from build123d import *

# Parameters (mm, degrees)
F1_DEPTH = 4
F0_W     = 28
F0_H     = 79
F2_DEPTH = 30
F3_W     = 10
F3_H     = 1.5
F4_DEPTH = 4
F6_DEPTH = 30
F5_W     = 20
F5_H     = 42
F7_DEPTH = 4
F8_R     = 5
F9_DEPTH = 4


with BuildPart() as f1:
    # F0 (on Top) → F1 (new body)
    with BuildSketch(Plane.XY):
        Polygon((17, 4), (24, 4), (24, 75), (4, 75), (4, 4), (11, 4), (11, 5.5), (14, 5.5), (17, 5.5), align=None)
    extrude(amount=F1_DEPTH)

    # F0 (on Top) → F2 (join)
    with BuildSketch(Plane.XY):
        with Locations((14, 39.5)):
            Rectangle(F0_W, F0_H)
        Polygon((24, 75), (24, 4), (17, 4), (14, 4), (11, 4), (4, 4), (4, 75), align=None, mode=Mode.SUBTRACT)
    extrude(amount=F2_DEPTH)

    # F3 (on face) → F4 (cut, through all)
    with BuildSketch(Plane(origin=(0, 79, 0), x_dir=(-1, 0, 0), z_dir=(0, 1, 0))):
        with Locations((-9, 29.25)):
            Rectangle(F3_W, F3_H)
        with Locations((-19, 29.25)):
            Rectangle(F3_W, F3_H)
    extrude(amount=-F4_DEPTH, mode=Mode.SUBTRACT)

    # F5 (on Top) → F6 (join)
    with BuildSketch(Plane.XY):
        Polygon((24, 79), (28, 79), (28, 125), (0, 125), (0, 79), (4, 79), (4, 121), (24, 121), align=None)
    extrude(amount=F6_DEPTH)

    # F5 (on Top) → F7 (join)
    with BuildSketch(Plane.XY):
        with Locations((14, 100)):
            Rectangle(F5_W, F5_H)
    extrude(amount=F7_DEPTH)

    # F8 (on face) → F9 (cut, through all)
    with BuildSketch(Plane(origin=(0, 125, 0), x_dir=(-1, 0, 0), z_dir=(0, 1, 0))):
        with Locations((-14, 15)):
            Circle(F8_R)
    extrude(amount=-F9_DEPTH, mode=Mode.SUBTRACT)


solid = f1.part
Model file for the job. Use its own axes, mm. A direction names the side the tool comes from. Give positions to 0.01 mm unless a question says otherwise; leave off trailing zeros. Order: outer loops, then holes, each group sorted by start corner. A loop starts at its lowest first (then second) coordinate and runs counter-clockwise, first axis right, second up. Notation, with made-up numbers: M 14.5,72.5 L 66.5,72.5 A25 ccw 66.5,97.5 Z; hole C 22,6 d7. An arc over 180 degrees is marked long. Put each result on its own line as item: value. Start each with the question number.
(1) Band-saw the part on D-D on z = 15. Give the cut face in (x, y).
(2) Band-saw the part on A-A on z = 21.75. Give the cut face in (x, y).
(3) Drill centre lines: L1, parallel to Y at x = 14.25, z = 8.25; L2, parallel to X at y = 12.5, z = 15.25; L3, parallel to Z at x = 14, y = 122.75. Where is each one in solid material? Low to high. Write a range as [from, to].
(4) Pin check, flat tips, straight feed: pin 1 Ø2 at (x, z) = (13.5, 17) entering from +Y; pin 2 Ø8 at (y, z) = (46, 12.5) entering from -X; pin 3 Ø4.5 at (x, y) = (14.5, 76) entering from +Z; pin 4 Ø3 at (x, y) = (16, 104.5) entering from +Z. Stop position of each tip, or through.
(5) Band-saw the part on C-C on y = 33.5. Give the cut face in (x, z).
(6) Tool access for faces 1 (the face through (0, 63, 15)), 2 (the face through (14, 5.5, 2)), 3 (the face through (14, 4, 15)): list every direction of +Z, -Z, +X, -X, +Y, -Y with a clear straight run to the whole face (end or side of a thin tool).
(7) Band-saw the part on B-B on x = 14. Give the cut face in (y, z).
(8) Pull direction Z, two halves, no side cores. Call faces 4 (the face through (11.693, 123.028, 10.564)), 5 (the face through (3.6, 58.2, 30)), 6 (the face through (14, 63, 0)), 7 (the face through (16, 121, 20)): released by +Z, released by -Z, zero draft, split by the parting line, or undercut.
Results below:
1. outline: M 0,0 L 28,0 L 28,125 L 19,125 L 19,121 L 24,121 L 24,79 L 4,79 L 4,121 L 9,121 L 9,125 L 0,125 Z; hole M 4,4 L 24,4 L 24,75 L 4,75 Z
2. outline: M 0,0 L 28,0 L 28,125 L 0,125 Z; hole M 4,4 L 24,4 L 24,75 L 4,75 Z; hole M 4,79 L 24,79 L 24,121 L 4,121 Z
3. L1: y = [0, 4], [75, 79], [121, 125]
3. L2: x = [0, 4], [24, 28]
3. L3: z = [0, 10], [20, 30]
4. pin 1: stops at y = 79
4. pin 2: stops at x = 0
4. pin 3: stops at z = 28.5
4. pin 4: stops at z = 4
5. outline: M 0,0 L 28,0 L 28,30 L 24,30 L 24,4 L 4,4 L 4,30 L 0,30 Z
6. face 1: +Z, -Z, -X, +Y, -Y
6. face 2: +Z, -Z
6. face 3: +Z
7. outline: M 0,0 L 4,0 L 4,30 L 0,30 Z; M 5.5,0 L 125,0 L 125,10 L 121,10 L 121,4 L 79,4 L 79,28.5 L 75,28.5 L 75,4 L 5.5,4 Z; M 121,20 L 125,20 L 125,30 L 121,30 Z
8. face 4: undercut
8. face 5: released by +Z
8. face 6: released by -Z
8. face 7: zero draft
